from build123d import *

# Parameters (mm, degrees)
BOSS_EXTRUDE1_DEPTH     = 600
SKETCH2_R               = 250
BOSS_EXTRUDE3_DEPTH     = 350
SKETCH6_R               = 200
CUT_EXTRUDE1_DEPTH      = 100
SKETCH8_R               = 100
SKETCH7_R               = 150
FILLET2_R               = 100
FILLET3_R               = 10
SKETCH11_R              = 58.235787107
CUT_EXTRUDE5_DEPTH      = 1362.628038628
CUT_EXTRUDE5_DEPTH_BACK = 1362.628038628
CUT_EXTRUDE6_REACH      = 1281.27
SKETCH12_R              = 70
RIB1_REACH              = 1260.583
SKETCH13_WALL_W         = 2854.575996278
SKETCH13_WALL_H         = 120
RIB2_REACH              = 1260.583
SKETCH14_WALL_W         = 2854.575996278
SKETCH14_WALL_H         = 120


with BuildPart() as part:
    # Sketch1 → Boss-Extrude1 (new body)
    with BuildSketch(Plane.XY):
        Polygon((-175.862068966, 0), (-575.862068966, 0), (-575.862068966, 150), (-325.862068966, 150), (-325.862068966, 450), (662.068965517, 450), (662.068965517, 150), (924.137931034, 150), (924.137931034, 0), (524.137931034, 0), (524.137931034, 300), (-175.862068966, 300), align=None)
    extrude(amount=BOSS_EXTRUDE1_DEPTH)

    # Sketch2 → Boss-Extrude3 (add)
    with BuildSketch(Plane(origin=(0, 450, 0), x_dir=(1, 0, 0), z_dir=(0, 1, 0))):
        with Locations(Location((174.137931034, -300, 0), (0, 0, 270))):
            Circle(SKETCH2_R)
    extrude(amount=BOSS_EXTRUDE3_DEPTH)

    # Sketch6 → Cut-Extrude1 (cut)
    with BuildSketch(Plane(origin=(0, 800, 0), x_dir=(1, 0, 0), z_dir=(0, 1, 0))):
        with Locations(Location((174.137931034, -300, 0), (0, 0, 270))):
            Circle(SKETCH6_R)
    extrude(amount=-CUT_EXTRUDE1_DEPTH, mode=Mode.SUBTRACT)

    # Sketch8 → Cut-Loft1 section 0
    with BuildSketch(Plane.XZ.offset(-300)):
        with Locations((174.137931034, 300)):
            Circle(SKETCH8_R)
    # Sketch7 → Cut-Loft1 section 1
    with BuildSketch(Plane(origin=(0, 700, 0), x_dir=(1, 0, 0), z_dir=(0, 1, 0))):
        with Locations((174.137931034, -300)):
            Circle(SKETCH7_R)
    loft(mode=Mode.SUBTRACT)

    # Fillet2
    fillet2_edges = [part.edges().sort_by_distance(p)[0] for p in [
        (-575.862068966, 75, 0),
        (-575.862068966, 75, 600),
    ]]
    fillet(fillet2_edges, radius=FILLET2_R)

    # Fillet3
    fillet3_edges = [part.edges().sort_by_distance(p)[0] for p in [
        (-325.862068966, 450, 300),
        (662.068965517, 450, 300),
    ]]
    fillet(fillet3_edges, radius=FILLET3_R)

    # Sketch11 → Cut-Extrude5 (cut, two sides)
    with BuildSketch(Plane.XY) as cut_extrude5_sk:
        with Locations(Location((174.137931034, 590, 0), (0, 0, 90.000000003))):
            Circle(SKETCH11_R)
    extrude(amount=CUT_EXTRUDE5_DEPTH, mode=Mode.SUBTRACT)
    extrude(cut_extrude5_sk.sketch, amount=-CUT_EXTRUDE5_DEPTH_BACK, mode=Mode.SUBTRACT)

    # Sketch12 → Cut-Extrude6 (cut, up to next)
    with BuildSketch(Plane(origin=(0, 150, 0), x_dir=(1, 0, 0), z_dir=(0, 1, 0)), mode=Mode.PRIVATE) as cut_extrude6_sk1:
        with Locations((924.137931034, -300)):
            Circle(SKETCH12_R)
    cut_extrude6_tool1 = extrude(cut_extrude6_sk1.sketch, amount=-CUT_EXTRUDE6_REACH, mode=Mode.PRIVATE) & part.part
    add(cut_extrude6_tool1.solids().sort_by_distance((924.137931, 150, 300))[0], mode=Mode.SUBTRACT)

    # Sketch13 wall → Rib1 (add, up to next)
    with BuildSketch(Plane(origin=(-100.862068966, 150, 300), x_dir=(0.4472135955, 0.894427191, 0), z_dir=(-0.894427191, 0.4472135955, 0)), mode=Mode.PRIVATE) as rib1_sk1:
        Rectangle(SKETCH13_WALL_W, SKETCH13_WALL_H)
    rib1_tool1 = extrude(rib1_sk1.sketch, amount=RIB1_REACH, mode=Mode.PRIVATE) - part.part
    add(rib1_tool1.solids().sort_by_distance((-100.862068966, 150, 300))[0])

    # Sketch14 wall → Rib2 (add, up to next)
    with BuildSketch(Plane(origin=(449.137931034, 150, 300), x_dir=(-0.4472135955, 0.894427191, 0), z_dir=(-0.894427191, -0.4472135955, 0)), mode=Mode.PRIVATE) as rib2_sk1:
        Rectangle(SKETCH14_WALL_W, SKETCH14_WALL_H)
    rib2_tool1 = extrude(rib2_sk1.sketch, amount=-RIB2_REACH, mode=Mode.PRIVATE) - part.part
    add(rib2_tool1.solids().sort_by_distance((449.137931034, 150, 300))[0])


solid = part.part
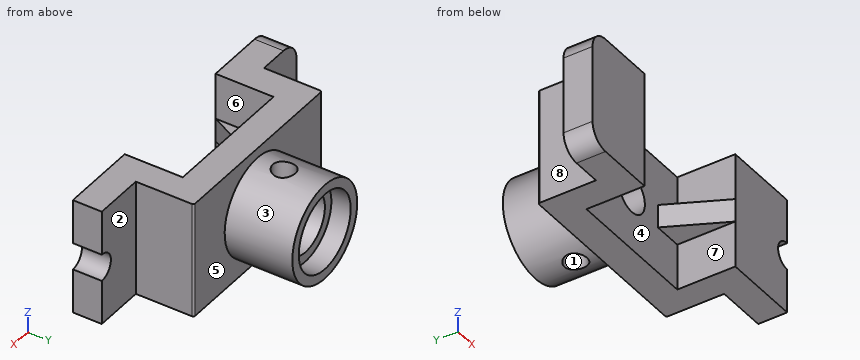
Check sheet for the modelled part. Datum: model origin and axes. Units: mm. Face numbers are marked on the shaded views. A direction names the side the tool comes from. Give positions to 0.01 mm unless a question says otherwise; leave off trailing zeros. Loops run counter-clockwise (first coordinate to the right, second up) from the corner with the lowest first, then second, coordinate; pieces in that order, holes last. Notation, with made-up numbers: M -9,-21 L 2,-21 A15 cw 2,-13 Z; hole C 39,36 d1. An arc over 180 degrees is marked long. Use a Markdown table: item, result. Add a question column.
Q1. Tool access check on the marked faces 4, 5, 6, 7 and 8. Record the directions out of +Z, -Z, +X, -X, +Y, -Y that give a thin tool (end or side, any length) a straight path to the whole face; none if there is none.
Q2. Sectioned sample at D-D, the plane x = 138.5. Give the number of separate pieces and of enclosed holes in the cut face, then the cut area to 3 significant figures.
Q3. Go/stop test with flat-tipped pins: pin 1 (5 mm diameter, centred on y = 306, z = 435, fed in from -X); pin 2 (6 mm diameter, centred on y = 296, z = 211.5, fed in from +X); pin 3 (1 mm diameter, centred on x = 113, y = 520, fed in from +Z). Record where each tip stops, or that it passes through.
Q4. Sectioned sample at B-B, the plane x = 704.5. Record the cut outline in (y, z), then the cut area to 3 significant figures.
Q5. Sectioned sample at A-A, the plane y = 632.5. Record the cut outline in (x, z) (1 decimal), then the cut area to 3 significant figures.
Q6. Sectioned sample at C-C, the plane y = 723.5. Record the cut outline in (x, z).
Q7. Scan lines: line 1 along X through (y, z) = (285, 428); line 2 along X through (y, z) = (726, 300); line 3 along Y through (x, z) = (-60.5, 397.5). Record each from-to range of solid material in increasing order. Write a range as [from, to].
Q8. Mould release check, pull along X, two halves, no side actions. Record for the marked faces 1, 2 and 3: pulls with the +X half, pulls with the -X half, needs draft (parallel to the pull), parting line crosses it, or undercut.
Verdict:
| question | item | result |
|---|---|---|
| 1 | face 4 | -Y |
| 1 | face 5 | +Y |
| 1 | face 6 | +Z, -Y |
| 1 | face 7 | -Z, -Y |
| 1 | face 8 | +Z, -Z, -X, +Y |
| 2 | separate pieces | 4 |
| 2 | enclosed holes | 0 |
| 2 | area | 107,000 mm^2 |
| 3 | pin 1 | x = -325.86 |
| 3 | pin 2 | x = 662.07 |
| 3 | pin 3 | z = 542.53 |
| 4 | outline | M 0,0 L 150,0 L 150,600 L 0,600 Z |
| 4 | area | 90,000 mm^2 |
| 5 | outline | M 134.3,53.2 L 134.3,164.2 A141.6 cw 134.3,435.8 L 134.3,546.8 A250 ccw Z; M 214,53.2 A250 ccw 214,546.8 L 214,435.8 A141.6 cw 214,164.2 Z |
| 5 | area | 116,000 mm^2 |
| 6 | outline | C 174.14,300 d500; hole C 174.14,300 d400 |
| 7 | line 1 | [-325.86, -175.86], [524.14, 662.07] |
| 7 | line 2 | [-75.86, -25.86], [374.14, 424.14] |
| 7 | line 3 | [300, 450] |
| 8 | face 1 | undercut |
| 8 | face 2 | needs draft |
| 8 | face 3 | parting line crosses it |
